from build123d import *

# Parameters (mm, degrees)
SKETCH_R     = 2.5
PAD_DEPTH    = 2.5
PAD001_DEPTH = 4.5
SKETCH002_R  = 1.5
PAD002_DEPTH = 14.2
POCKET_DEPTH = 10


with BuildPart() as part:
    # Sketch → Pad (new body)
    with BuildSketch(Plane.XY):
        Polygon((19.5, 5.5), (19.5, -5.5), (5, -5.5), (5, -8.641544), (-5, -8.641544), (-5, -5.5), (-19.5, -5.5), (-19.5, 5.5), (-8.5, 5.5), (-8.5, 5.6), (-5.6, 5.6), (-5.6, 5.5), (-5.5, 5.5), (-5.5, 2.5), (5.5, 2.5), (5.5, 5.5), (5.6, 5.5), (5.6, 5.6), (8.5, 5.6), (8.5, 5.5), align=None)
        with Locations((-8.25, 0)):
            Circle(SKETCH_R, mode=Mode.SUBTRACT)
        with Locations((8.25, 0)):
            Circle(SKETCH_R, mode=Mode.SUBTRACT)
    extrude(amount=PAD_DEPTH)

    # Sketch001 (on Face24 of Pad) → Pad001 (join)
    with BuildSketch(Plane.XY.offset(2.5)):
        with BuildLine():
            Line((5.6, 5.6), (5.6, 8.6))
            Line((5.6, 8.6), (7.1, 8.6))
            Line((7.1, 8.6), (7.1, 2.6))
            ThreePointArc((7.1, 2.6), (5.590571, 1.671077), (5, 0))
            Line((5, -8.641543), (5, 0))
            Line((3.5, -8.641543), (5, -8.641543))
            Line((3.5, 2.5), (3.5, -8.641543))
            Line((5.6, 2.5), (3.5, 2.5))
            Line((5.6, 5.6), (5.6, 2.5))
        make_face()
        with BuildLine():
            Line((-7.1, 8.6), (-5.6, 8.6))
            Line((-5.6, 8.6), (-5.6, 2.5))
            Line((-5.6, 2.5), (-3.5, 2.5))
            Line((-3.5, 2.5), (-3.5, -8.641543))
            Line((-3.5, -8.641543), (-5, -8.641543))
            Line((-5, -8.641543), (-5, 0))
            ThreePointArc((-5, 0), (-5.590571, 1.671077), (-7.1, 2.6))
            Line((-7.1, 2.6), (-7.1, 8.6))
        make_face()
    extrude(amount=PAD001_DEPTH)

    # Sketch002 (on Face44 of Pad001) → Pad002 (join)
    with BuildSketch(Plane.YZ.offset(7.1)):
        with Locations((6.7, 4.5)):
            Circle(SKETCH002_R)
    extrude(amount=-PAD002_DEPTH)

    # Sketch003 (on Face35 of Pad002) → Pocket (cut)
    with BuildSketch(Plane(origin=(-5, 0, 0), x_dir=(0, -1, 0), z_dir=(-1, 0, 0))):
        with BuildLine():
            ThreePointArc((4.426559, 5.882108), (4.923015, 2.847853), (7.20048, 4.913363))
            Line((7.20048, 4.913363), (7.655942, 7.49642))
            Line((4.8, 8), (7.655942, 7.49642))
            Line((4.8, 8), (4.426559, 5.882108))
        make_face()
    extrude(amount=-POCKET_DEPTH, mode=Mode.SUBTRACT)


solid = part.part
Model file for the job. Use its own axes, mm. A direction names the side the tool comes from. Give positions to 0.01 mm unless a question says otherwise; leave off trailing zeros. Order: outer loops, then holes, each group sorted by start corner. A loop starts at its lowest first (then second) coordinate and runs counter-clockwise, first axis right, second up. Notation, with made-up numbers: (-8, 83.25) - (1, 83.25) arc R19 ccw to (1, 91.25) - close; hole circle Ø11 at (-9, 73). An arc over 180 degrees is marked (long way). One line per item, written item: value.
Item 1: Pin check, flat tips, straight feed: pin 1 Ø0.8 at (x, z) = (7, 1) entering from +Y; pin 2 Ø1 at (x, z) = (1.5, 5.5) entering from -Y; pin 3 Ø1.6 at (x, y) = (-6.5, 6.5) entering from -Z; pin 4 Ø3.5 at (y, z) = (-5, 3) entering from +X. Stop position of each tip, or through.
Response values:
pin 1: y = 5.6
pin 2: y = 5.29
pin 3: z = 2.5
pin 4: x = 19.5
Item 2: Wall check: line 1 (X direction, y = -1, z = 4.75); line 2 (Y direction, x = -8.25, z = 1.15); line 3 (X direction, y = 3.5, z = 4.25). Give the ranges that are in metal, low to high.
Response values:
line 1: -5 to -3.5, 3.5 to 5
line 2: -5.5 to -2.5, 2.5 to 5.6
line 3: -7.1 to -5.6, 5.6 to 7.1
Item 3: Slice it at A-A (z = 4.5). List the corners of the cut face in (x, y), then the cut area to 3 significant figures.
Response values:
outline: (-7.1, 2.6) arc R2.66 cw to (-5, 0) - (-5, -3.75) - (-3.5, -3.75) - (-3.5, 2.5) - (-5.6, 2.5) - (-5.6, 5.2) - (5.6, 5.2) - (5.6, 2.5) - (3.5, 2.5) - (3.5, -3.75) - (5, -3.75) - (5, 0) arc R2.66 cw to (7.1, 2.6) - (7.1, 8.6) - (5.6, 8.6) - (5.6, 8.2) - (-5.6, 8.2) - (-5.6, 8.6) - (-7.1, 8.6) - close; (-5, -8.64) - (-3.5, -8.64) - (-3.5, -7.25) - (-5, -7.25) - close; (3.5, -8.64) - (5, -8.64) - (5, -7.25) - (3.5, -7.25) - close
area: 77.2 mm2
Item 4: Slice it at B-B (x = -0.5). List the corners of the cut face in (y, z).
Response values:
outline: (-8.64, 0) - (2.5, 0) - (2.5, 2.5) - (-8.64, 2.5) - close; circle Ø3 at (6.7, 4.5)
Item 5: Slice it at D-D (y = 6.7). List the corners of the cut face in (x, z).
Response values:
outline: (-7.1, 2.5) - (-5.6, 2.5) - (-5.6, 3) - (5.6, 3) - (5.6, 2.5) - (7.1, 2.5) - (7.1, 7) - (5.6, 7) - (5.6, 6) - (-5.6, 6) - (-5.6, 7) - (-7.1, 7) - close
Item 6: Tool access for faces 1 (the flat face through (-5.6, 5, 4)), 2 (the flat face through (7.1, 6, 5)), 3 (the flat face through (7, 5.6, 1)), 4 (the cylindrical face through (5.607, 1.691, 4.719)): list every direction of +Z, -Z, +X, -X, +Y, -Y with a clear straight run to the whole face (end or side of a thin tool).
Response values:
face 1: none
face 2: +Z, +X, +Y, -Y
face 3: -Z, +X, -X, +Y
face 4: +Z, +X, -Y
Item 7: Slice it at C-C (z = 1.75). List the corners of the cut face in (x, y), then the cut area to 3 significant figures.
Response values:
outline: (-19.5, -5.5) - (-5, -5.5) - (-5, -8.64) - (5, -8.64) - (5, -5.5) - (19.5, -5.5) - (19.5, 5.5) - (8.5, 5.5) - (8.5, 5.6) - (5.6, 5.6) - (5.6, 5.5) - (5.5, 5.5) - (5.5, 2.5) - (-5.5, 2.5) - (-5.5, 5.5) - (-5.6, 5.5) - (-5.6, 5.6) - (-8.5, 5.6) - (-8.5, 5.5) - (-19.5, 5.5) - close; hole circle Ø5 at (-8.25, 0); hole circle Ø5 at (8.25, 0)
area: 389 mm2
Item 8: Two-plate mould, pull along Y, no slides. Class faces 5 (the flat face through (12, -5.5, 1)), 6 (the flat face through (-14, 5.5, 1)), 7 (the flat face through (-4.26, -7.38, 5.94)): released by +Y, released by -Y, zero draft, split by the parting line, or undercut.
Response values:
face 5: released by -Y
face 6: released by +Y
face 7: undercut
